```python
from build123d import *

# Parameters (mm, degrees)
SKETCH1_R           = 1.5
BOSS_EXTRUDE1_DEPTH = 6
SKETCH2_R           = 1
BOSS_EXTRUDE2_DEPTH = 2
FILLET1_R           = 1
SKETCH3_R           = 0.5
BOSS_EXTRUDE3_DEPTH = 50


with BuildPart() as part:
    # Sketch1 → Boss-Extrude1 (new body)
    with BuildSketch(Plane(origin=(0, 0, 0), x_dir=(1, 0, 0), z_dir=(0, 1, 0))):
        with Locations(Location((0, 0, 0), (0, 0, 270))):
            Circle(SKETCH1_R)
    extrude(amount=BOSS_EXTRUDE1_DEPTH)

    # Sketch2 → Boss-Extrude2 (add)
    with BuildSketch(Plane(origin=(0, 6, 0), x_dir=(1, 0, 0), z_dir=(0, 1, 0))):
        with Locations(Location((0, 0, 0), (0, 0, 270))):
            Circle(SKETCH2_R)
    extrude(amount=BOSS_EXTRUDE2_DEPTH)

    # Fillet1
    # the kernel refuses this fillet: 1 mm, written as the material it adds along each edge
    with BuildSketch(Plane(origin=(0, 6, 0), x_dir=(0, 0, 1), z_dir=(-1, 0, 0))) as fillet1_piece_1:
        with BuildLine():
            CenterArc((2, 0.866025404), FILLET1_R, 180, 60)
            Line((1, 0.866025404), (0.98, 0.866025404))
            Line((0.98, 0.866025404), (0.98, 0))
            Line((0.98, 0), (1, -0.02))
            ThreePointArc((1, -0.02), (1.25, -0.02), (1.49, -0.017320508))
            Line((1.49, -0.017320508), (1.5, 0))
        make_face()
    revolve(axis=Axis((0, 6, 0), (0, 1, 0)))

    # Sketch3 → Boss-Extrude3 (add)
    with BuildSketch(Plane(origin=(0, 8, 0), x_dir=(1, 0, 0), z_dir=(0, 1, 0))):
        with Locations(Location((0, 0, 0), (0, 0, 270))):
            Circle(SKETCH3_R)
    extrude(amount=BOSS_EXTRUDE3_DEPTH)


solid = part.part
```
The model under review builds one solid part; all positions refer to its coordinate system, in mm. A direction names the side the tool comes from. Round coordinates to 2 decimals unless told otherwise and drop trailing zeros. Write each loop counter-clockwise with the first axis right and the second up, starting at its lowest first coordinate (ties: lowest second). Pieces come first, ordered by that corner, then holes. Notation, with made-up numbers: (69.25, 53.25) - (127.25, 53.25) arc R12 cw to (127.25, 57.25) - close; hole circle Ø1 at (61, 57.5). An arc over 180 degrees is marked (long way). Answer as CSV lines item,"result". Start each with the question number.
(1) For pin 1 Ø1.5 at (y, z) = (49, -0.5) entering from -X, flat-tipped, find the tip position at first contact; note if it passes through.
(2) To check wall thickness, follow line 1 (Y direction, x = 0.5, z = -0.6); line 2 (Z direction, x = 0.1, y = 45); line 3 (X direction, y = 5, z = 0.1). State the ranges of each line that lie inside material, in increasing order.
(3) We need section D-D on y = 7.5. State the section outline as (x, z) points, plus the area to 3 significant figures.
(4) We need section C-C on y = 19. State the section outline as (x, z) points, plus the area to 3 significant figures.
(5) We need section B-B on x = 0. State the section outline as (y, z) points.
(6) We need section A-A on z = 0. State the section outline as (x, y) points.
(7) For faces 1 (the flat face through (0, 58, 0)), 2 (the cylindrical face through (-0.488, 32.65, -0.108)), list the 3-axis set-ups (+Z, -Z, +X, -X, +Y, -Y) from which the entire face can be reached by the end or side of a thin tool; tool diameter is ignored.
Worked answers:
1,pin 1,"x = -0.5"
2,line 1,"0 to 8"
2,line 2,"-0.49 to 0.49"
2,line 3,"-1.5 to 1.5"
3,outline,"circle Ø2 at (0, 0)"
3,area,"3.14 mm²"
4,outline,"circle Ø1 at (0, 0)"
4,area,"0.785 mm²"
5,outline,"(0, -1.5) - (6, -1.5) arc R1 cw to (6.87, -1) - (8, -1) - (8, -0.5) - (58, -0.5) - (58, 0.5) - (8, 0.5) - (8, 1) - (6.87, 1) arc R1 cw to (6, 1.5) - (0, 1.5) - close"
6,outline,"(-1.5, 0) - (1.5, 0) - (1.5, 6) arc R1 cw to (1, 6.87) - (1, 8) - (0.5, 8) - (0.5, 58) - (-0.5, 58) - (-0.5, 8) - (-1, 8) - (-1, 6.87) arc R1 cw to (-1.5, 6) - close"
7,face 1,"+Z, -Z, +X, -X, +Y"
7,face 2,"+Y"
